Could you check a few things on this drawing? It's one solid part, dimensions in mm from its lowest x, y, z. Coordinates: 2 decimals unless noted, no trailing zeros. Write each loop counter-clockwise with the first axis right and the second up, starting at its lowest first coordinate (ties: lowest second). Pieces come first, ordered by that corner, then holes. Notation, with made-up numbers: (70.5, 2) - (84.5, 2) arc R5 cw to (84.5, 6) - close; hole circle Ø6 at (-22, 8). An arc over 180 degrees is marked (long way). Use one line per item in the form item = value. Start each with the question number.
(1) For pin 1 Ø5.5 at (x, z) = (6, 4.5) entering from -Y; pin 2 Ø9 at (y, z) = (60.5, 10.5) entering from +X; pin 3 Ø5.5 at (y, z) = (330, 7) entering from -X, each with a flat end and sliding along its axis, tell me the tip position at first contact or that it passes through.
(2) If we section it at B-B on z = 13.5: Please give me the cut outline in (x, y), then the cut area to 3 significant figures.
(3) If we section it at C-C on y = 462: Please give me the cut outline in (x, z).
(4) If we section it at A-A on y = 261: Please give me the cut outline in (x, z), then the cut area to 3 significant figures.
(5) If I drill on probe 1 along X at (y, z) = (398, 11.75); probe 2 along X at (y, z) = (204, 1); probe 3 along X at (y, z) = (30.5, 7), over which ranges is the centre line in solid material (lowest first)? Write a range as from..to.
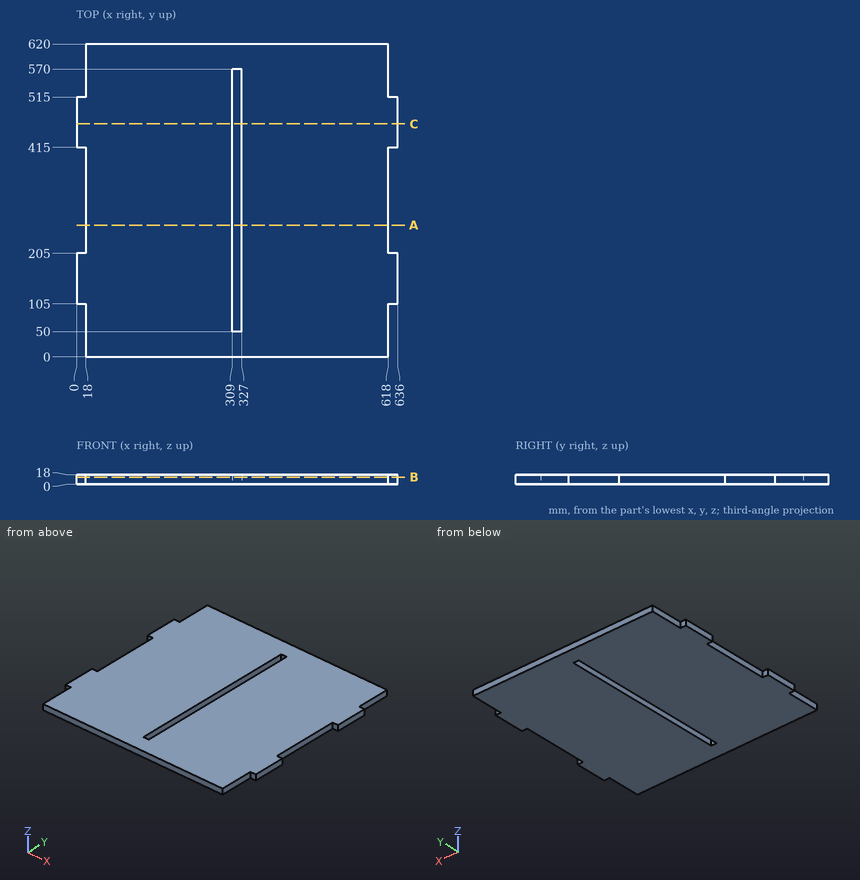
Reported:
q1.pin_1 = 105
q1.pin_2 = 618
q1.pin_3 = 18
q2.outline = (0, 105) - (18, 105) - (18, 0) - (618, 0) - (618, 105) - (636, 105) - (636, 205) - (618, 205) - (618, 415) - (636, 415) - (636, 515) - (618, 515) - (618, 620) - (18, 620) - (18, 515) - (0, 515) - (0, 415) - (18, 415) - (18, 205) - (0, 205) - close; hole (309, 50) - (327, 50) - (327, 570) - (309, 570) - close
q2.area = 370,000 mm2
q3.outline = (0, 0) - (309, 0) - (309, 18) - (0, 18) - close; (327, 0) - (636, 0) - (636, 18) - (327, 18) - close
q4.outline = (18, 0) - (309, 0) - (309, 18) - (18, 18) - close; (327, 0) - (618, 0) - (618, 18) - (327, 18) - close
q4.area = 10,500 mm2
q5.probe_1 = 18..309, 327..618
q5.probe_2 = 0..309, 327..636
q5.probe_3 = 18..618
